The listing builds one solid part. Answer for the finished solid, in the listing's coordinates (mm). Face numbers are marked on the shaded views. A direction names the side the tool comes from. Coordinates: 2 decimals unless noted, no trailing zeros. Order: outer loops, then holes, each group sorted by start corner. A loop starts at its lowest first (then second) coordinate and runs counter-clockwise, first axis right, second up. Notation, with made-up numbers: (-11.5, 34.5) - (44.5, 34.5) arc R7 cw to (44.5, 40.5) - close; hole circle Ø5 at (21.25, 4.25). An arc over 180 degrees is marked (long way). Use a Markdown table: item, result. Add a question column.
Item 1: The part is cut by section A-A, the plane y = 18. Give the vertices of the cut face in (x, z), then the cut area to 3 significant figures.
Item 2: The part is cut by section D-D, the plane x = -23.5. Give the vertices of the cut face in (y, z).
Item 3: Find the intervals of material crossed by line 1 along X through (y, z) = (18, 55); line 2 along Z through (x, y) = (-5.5, 51); line 3 along X through (y, z) = (51, 51.5), in increasing order.
Item 4: The part is cut by section C-C, the plane z = 51. Give the vertices of the cut face in (x, y), then the cut area to 3 significant figures.
Item 5: The mould has two halves that part along Z. Classify the marked faces 1, 2, 3 and 4: released by +Z, released by -Z, zero draft, split by the parting line, or undercut.
Item 6: Flat-ended cylindrical pins translate along their axes: P1, Ø10, axis at x = -6, z = 9, coming from the +Y side; P2, Ø15.5, axis at x = -36, z = 5.5, coming from the +Y side; P3, Ø10, axis at y = 8, z = 34, coming from the -X side; P4, Ø14.5, axis at x = -29.53, y = 18, coming from the -Z side. Find the tip coordinate at first contact, or state that the pin passes through.
Item 7: The part is cut by section B-B, the plane x = 27.5. Give the vertices of the cut face in (y, z).
Item 8: For the marked faces 5, 6, 7 and 8, determine the directions among +Z, -Z, +X, -X, +Y, -Y from which every point of the face is accessible in a straight line to the end or side of a thin tool.
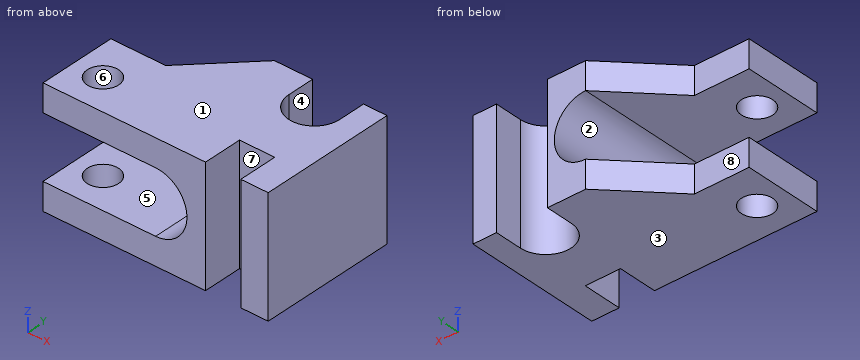
from build123d import *

# Parameters (mm, degrees)
SKETCH1_R           = 8
BOSS_EXTRUDE1_DEPTH = 60
CUT_EXTRUDE1_DEPTH  = 117.040965384


with BuildPart() as part:
    # Sketch1 → Boss-Extrude1 (new body)
    # profile 1 of 2: a face of its own
    with BuildSketch(Plane.XY):
        with BuildLine():
            Line((12.966344075, 70), (12.966344075, 0))
            Line((12.966344075, 0), (38.466344075, 0))
            Line((38.466344075, 0), (38.466344075, 20))
            Line((38.466344075, 20), (56.466344075, 20))
            Line((56.466344075, 20), (56.466344075, 0))
            Line((56.466344075, 0), (70.466344075, 0))
            Line((70.466344075, 0), (70.466344075, 70))
            Line((70.466344075, 70), (58.466344075, 70))
            Line((58.466344075, 70), (58.466344075, 56))
            ThreePointArc((58.466344075, 56), (45.466344075, 43), (32.466344075, 56))
            Line((32.466344075, 56), (32.466344075, 70))
            Line((32.466344075, 70), (12.966344075, 70))
        make_face()
    # profile 2 of 2: a face of its own
    with BuildSketch(Plane.XY):
        Polygon((-44.533655925, 0), (0, 0), (12.966344075, 0), (12.966344075, 70), (-16.533655925, 40), (-44.533655925, 40), align=None)
        with Locations((-29.533655925, 18)):
            Circle(SKETCH1_R, mode=Mode.SUBTRACT)
    extrude(amount=BOSS_EXTRUDE1_DEPTH)

    # Sketch2 → Cut-Extrude1 (cut, through all)
    with BuildSketch(Plane(origin=(0, 70, 0), x_dir=(1, 0, 0), z_dir=(0, 1, 0))):
        with BuildLine():
            Line((12.966344075, -14), (-56.308501396, -14))
            Line((-56.308501396, -14), (-56.308501396, -46))
            Line((-56.308501396, -46), (12.966344075, -46))
            ThreePointArc((12.966344075, -46), (28.966344075, -30), (12.966344075, -14))
        make_face()
    extrude(amount=-CUT_EXTRUDE1_DEPTH, mode=Mode.SUBTRACT)


solid = part.part
Solution:
| question | item | result |
|---|---|---|
| 1 | outline | (-44.53, 0) - (-37.53, 0) - (-37.53, 14) - (-44.53, 14) - close; (-44.53, 46) - (-37.53, 46) - (-37.53, 60) - (-44.53, 60) - close; (-21.53, 0) - (38.47, 0) - (38.47, 60) - (-21.53, 60) - (-21.53, 46) - (12.97, 46) arc R16 cw to (12.97, 14) - (-21.53, 14) - close; (56.47, 0) - (70.47, 0) - (70.47, 60) - (56.47, 60) - close |
| 1 | area | 3,130 mm2 |
| 2 | outline | (0, 0) - (12.75, 0) - (12.75, 14) - (0, 14) - close; (0, 46) - (12.75, 46) - (12.75, 60) - (0, 60) - close; (23.25, 0) - (40, 0) - (40, 14) - (23.25, 14) - close; (23.25, 46) - (40, 46) - (40, 60) - (23.25, 60) - close |
| 3 | line 1 | x = -44.53 to -37.53, -21.53 to 38.47, 56.47 to 70.47 |
| 3 | line 2 | z = 0 to 14, 46 to 60 |
| 3 | line 3 | x = -5.72 to 33.47, 57.47 to 70.47 |
| 4 | outline | (-44.53, 0) - (38.47, 0) - (38.47, 20) - (56.47, 20) - (56.47, 0) - (70.47, 0) - (70.47, 70) - (58.47, 70) - (58.47, 56) arc R13 cw to (32.47, 56) - (32.47, 70) - (12.97, 70) - (-16.53, 40) - (-44.53, 40) - close; hole circle Ø16 at (-29.53, 18) |
| 4 | area | 5,580 mm2 |
| 5 | face 1 | released by +Z |
| 5 | face 2 | undercut |
| 5 | face 3 | released by -Z |
| 5 | face 4 | zero draft |
| 6 | P1 | stops at y = 55.8 |
| 6 | P2 | stops at y = 40 |
| 6 | P3 | stops at x = 26.2 |
| 6 | P4 | passes through |
| 7 | outline | (0, 0) - (70, 0) - (70, 23.31) - (0, 23.31) - close; (0, 36.69) - (70, 36.69) - (70, 60) - (0, 60) - close |
| 8 | face 5 | -X, +Y, -Y |
| 8 | face 6 | +Z, -Z |
| 8 | face 7 | +Z, -Z, -Y |
| 8 | face 8 | +Z, -Z, -X, +Y |
